```python
from build123d import *

# Parameters (mm, degrees)
F1_DEPTH = 3
F2_DEPTH = 5
F4_DEPTH = 3


with BuildPart() as f1:
    # F0 (on Top) → F1 (new body)
    with BuildSketch(Plane.XY):
        Polygon((7, -60), (10, -60), (10, -10), (60, -10), (60, -7), (7, -7), align=None)
        Polygon((-7, -60), (7, -60), (7, -7), (60, -7), (60, 7), (7, 7), (7, 60), (-7, 60), (-7, 7), (-60, 7), (-60, -7), (-7, -7), align=None)
        Polygon((-10, -60), (-7, -60), (-7, -7), (-60, -7), (-60, -10), (-10, -10), align=None)
        Polygon((7, 7), (60, 7), (60, 10), (10, 10), (10, 60), (7, 60), align=None)
        Polygon((-60, 10), (-60, 7), (-7, 7), (-7, 60), (-10, 60), (-10, 10), align=None)
    extrude(amount=F1_DEPTH)

    # F0 (on Top) → F2 (join)
    with BuildSketch(Plane.XY):
        Polygon((7, 7), (60, 7), (60, 10), (10, 10), (10, 60), (7, 60), align=None)
        Polygon((-60, 10), (-60, 7), (-7, 7), (-7, 60), (-10, 60), (-10, 10), align=None)
        Polygon((-10, -60), (-7, -60), (-7, -7), (-60, -7), (-60, -10), (-10, -10), align=None)
        Polygon((7, -60), (10, -60), (10, -10), (60, -10), (60, -7), (7, -7), align=None)
    extrude(amount=-F2_DEPTH)

    # F3 (on face) → F4 (join)
    with BuildSketch(Plane(origin=(0, 0, -5), x_dir=(1, 0, 0), z_dir=(0, 0, -1))):
        Polygon((-4, 60), (-10, 60), (-10, 10), (-60, 10), (-60, 4), (-10, 4), (-4, 4), (-4, 10), align=None)
        Polygon((10, 10), (10, 60), (4, 60), (4, 10), (4, 4), (10, 4), (60, 4), (60, 10), align=None)
        Polygon((60, -4), (10, -4), (4, -4), (4, -10), (4, -60), (10, -60), (10, -10), (60, -10), align=None)
        Polygon((-10, -10), (-10, -60), (-4, -60), (-4, -10), (-4, -4), (-10, -4), (-60, -4), (-60, -10), align=None)
    extrude(amount=F4_DEPTH)


solid = f1.part
```
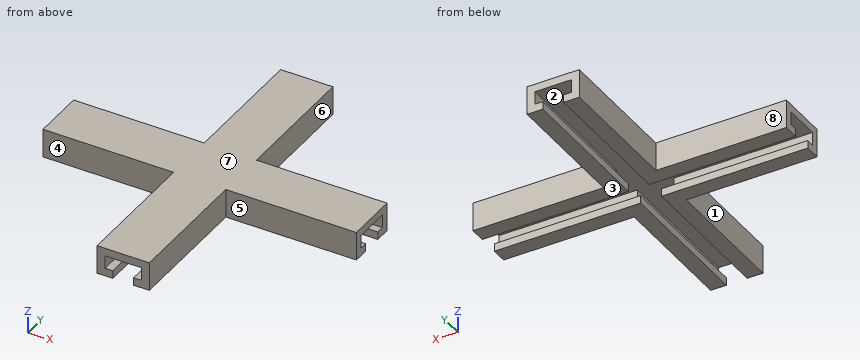
Check sheet for the modelled part. Datum: model origin and axes. Units: mm. Face numbers are marked on the shaded views. A direction names the side the tool comes from. Round coordinates to 2 decimals unless told otherwise and drop trailing zeros. Write each loop counter-clockwise with the first axis right and the second up, starting at its lowest first coordinate (ties: lowest second). Pieces come first, ordered by that corner, then holes. Notation, with made-up numbers: M 78.25,62 L 88.25,62 A30 cw 88.25,100 Z; hole C 61,-25.75 d7. An arc over 180 degrees is marked long. Write item = value, one per line. Start each with the question number.
1. Tool access check on the marked faces 4, 5, 6, 7 and 8. Record the directions out of +Z, -Z, +X, -X, +Y, -Y that give a thin tool (end or side, any length) a straight path to the whole face; none if there is none.
2. Gauge pin test, flat ends, axial feed: pin 1 (2.5 mm diameter, centred on y = 41, z = -6.5, fed in from -X); pin 2 (6 mm diameter, centred on x = 21.5, z = -0.5, fed in from -Y); pin 3 (5.5 mm diameter, centred on x = -32, z = -3, fed in from +Y). Record the tip position at first contact, or that the pin passes through.
3. Section check B-B, the plane y = 27. Record the cut outline in (x, z).
4. Section check A-A, the plane z = -2.5. Record the cut outline in (x, y).
5. Release check for a two-part mould opening along X. For the marked faces 1, 2 and 3 record: pulls with the +X half, pulls with the -X half, needs draft (parallel to the pull), parting line crosses it, or undercut.
6. Scan lines: line 1 (Z direction, x = 6, y = -37.5); line 2 (Y direction, x = 25, z = -0.25); line 3 (X direction, y = 5.5, z = -7.5). Record each from-to range of solid material in increasing order. Write a range as [from, to].
Results found:
q1.face_4 = +Z, -Z, -X, -Y
q1.face_5 = +Z, -Z, +X, -Y
q1.face_6 = +Z, -Z, +X, +Y
q1.face_7 = +Z, +X, -X, +Y, -Y
q1.face_8 = +Z, -Z, -X, +Y
q2.pin_1 = -10
q2.pin_2 = -10
q2.pin_3 = 10
q3.outline = M -10,-8 L -4,-8 L -4,-5 L -7,-5 L -7,0 L 7,0 L 7,-5 L 4,-5 L 4,-8 L 10,-8 L 10,3 L -10,3 Z
q4.outline = M -60,-10 L -10,-10 L -10,-60 L -7,-60 L -7,-7 L -60,-7 Z; M -60,7 L -7,7 L -7,60 L -10,60 L -10,10 L -60,10 Z; M 7,-60 L 10,-60 L 10,-10 L 60,-10 L 60,-7 L 7,-7 Z; M 7,7 L 60,7 L 60,10 L 10,10 L 10,60 L 7,60 Z
q5.face_1 = pulls with the -X half
q5.face_2 = undercut
q5.face_3 = needs draft
q6.line_1 = [-8, -5], [0, 3]
q6.line_2 = [-10, -7], [7, 10]
q6.line_3 = [-60, -4], [4, 60]
